from build123d import *

# Parameters (mm, degrees)
SKETCH_1_W             = 47.4
SKETCH_1_H             = 66.4
EXTRUDE_1_DEPTH        = 10
FILLET_1_R             = 3
FILLET_2_R             = 2
FILLET_4_R             = 1
FILLET_5_R             = 1
FILLET_1_OF_MIRROR_1_R = 3
FILLET_2_OF_MIRROR_1_R = 2
FILLET_4_OF_MIRROR_1_R = 1


with BuildPart() as part:
    # 草图1 → 凸台-拉伸1 (new body)
    with BuildSketch(Plane.XY):
        with BuildLine():
            ThreePointArc((-165.866679255, 23.5), (-260, 0), (-165.866679255, -23.5))
            Line((-165.866679255, -23.5), (0, -23.5))
            Line((0, -23.5), (0, 23.5))
            Line((0, 23.5), (-165.866679255, 23.5))
        make_face()
        with BuildLine():
            ThreePointArc((-187.901131251, -39.2), (-210, -45), (-232.098868749, -39.2))
            Line((-232.098868749, -39.2), (-187.901131251, -39.2))
        make_face(mode=Mode.SUBTRACT)
        with BuildLine():
            ThreePointArc((-239.7, -33.806951948), (-255, 0), (-239.7, 33.806951948))
            Line((-239.7, 33.806951948), (-239.7, -33.806951948))
        make_face(mode=Mode.SUBTRACT)
        with Locations((-210, 0)):
            Rectangle(SKETCH_1_W, SKETCH_1_H, mode=Mode.SUBTRACT)
        with BuildLine():
            Line((-187.901131251, 39.2), (-232.098868749, 39.2))
            ThreePointArc((-232.098868749, 39.2), (-210, 45), (-187.901131251, 39.2))
        make_face(mode=Mode.SUBTRACT)
    extrude_1 = extrude(amount=EXTRUDE_1_DEPTH)

    # 圆角1
    fillet_1_edges = [part.edges().sort_by_distance(p)[0] for p in [
        (-186.3, 33.2, 5),
        (-233.7, 33.2, 5),
        (-233.7, -33.2, 5),
        (-186.3, -33.2, 5),
    ]]
    fillet(fillet_1_edges, radius=FILLET_1_R)

    # 圆角2
    fillet_2_edges = [part.edges().sort_by_distance(p)[0] for p in [
        (-239.7, 33.806951948, 5),
        (-239.7, -33.806951948, 5),
    ]]
    fillet(fillet_2_edges, radius=FILLET_2_R)

    # 圆角4
    fillet_4_edges = [part.edges().sort_by_distance(p)[0] for p in [
        (-187.901131251, 39.2, 5),
        (-232.098868749, 39.2, 5),
        (-187.901131251, -39.2, 5),
        (-232.098868749, -39.2, 5),
    ]]
    fillet(fillet_4_edges, radius=FILLET_4_R)

    # 圆角5
    fillet_5_edges = [part.edges().sort_by_distance(p)[0] for p in [
        (-260, 0, 10),
        (-260, 0, 0),
    ]]
    fillet(fillet_5_edges, radius=FILLET_5_R)

    # 镜向1: 凸台-拉伸1 across plane
    add(extrude_1.mirror(Plane(origin=(0, 0, 10), x_dir=(0, 0, 1), z_dir=(1, 0, 0))))

    # 圆角1 of 镜向1
    fillet_1_of_mirror_1_edges = [part.edges().sort_by_distance(p)[0] for p in [
        (186.3, 33.2, 5),
        (233.7, 33.2, 5),
        (233.7, -33.2, 5),
        (186.3, -33.2, 5),
    ]]
    fillet(fillet_1_of_mirror_1_edges, radius=FILLET_1_OF_MIRROR_1_R)

    # 圆角2 of 镜向1
    fillet_2_of_mirror_1_edges = [part.edges().sort_by_distance(p)[0] for p in [
        (239.7, 33.806951948, 5),
        (239.7, -33.806951948, 5),
    ]]
    fillet(fillet_2_of_mirror_1_edges, radius=FILLET_2_OF_MIRROR_1_R)

    # 圆角4 of 镜向1
    fillet_4_of_mirror_1_edges = [part.edges().sort_by_distance(p)[0] for p in [
        (187.901131251, 39.2, 5),
        (232.098868749, 39.2, 5),
        (187.901131251, -39.2, 5),
        (232.098868749, -39.2, 5),
    ]]
    fillet(fillet_4_of_mirror_1_edges, radius=FILLET_4_OF_MIRROR_1_R)


solid = part.part
Geometry check sheet. Reference: the model listing, model coordinates, mm. A direction names the side the tool comes from. Give positions to 0.01 mm unless a question says otherwise; leave off trailing zeros. Order: outer loops, then holes, each group sorted by start corner. A loop starts at its lowest first (then second) coordinate and runs counter-clockwise, first axis right, second up. Notation, with made-up numbers: M 42,51.25 L 53,51.25 A8 cw 53,64.25 Z; hole C 16.5,-14 d11. An arc over 180 degrees is marked long. Use a Markdown table: item, result.
Item 1: Draft check along Y on faces 3 (the cylindrical face through (-259.966, 1.856, 4.944)), 4 (the flat face through (-186.3, 0, 5)), 5 (the flat face through (-239.7, 0, 5)), 6 (the flat face through (-3, 23.5, 5)). Enter one of: +Y half, -Y half, draft (parallel to the pull), parting line (faces both ways), or undercut.
Answers follow:
| item | result |
|---|---|
| face 3 | parting line |
| face 4 | undercut |
| face 5 | undercut |
| face 6 | +Y half |
Item 2: Depth check by flat-ended pin: P1, Ø4, axis at x = 48.5, z = 3, coming from the +Y side; P2, Ø3, axis at y = 12, z = 5.5, coming from the -X side; P3, Ø3, axis at y = 4.5, z = 5.5, coming from the -X side. Enter the tip coordinate at first touch or a pass-through.
Answers follow:
| item | result |
|---|---|
| P1 | stops at y = 23.5 |
| P2 | stops at x = -258.89 |
| P3 | stops at x = -259.91 |
Item 3: Section check B-B (x = 210). Record the cut outline in (y, z).
Answers follow:
| item | result |
|---|---|
| outline | M -50,0 L -45,0 L -45,10 L -50,10 Z; M -39.2,0 L -33.2,0 L -33.2,10 L -39.2,10 Z; M 33.2,0 L 39.2,0 L 39.2,10 L 33.2,10 Z; M 45,0 L 50,0 L 50,10 L 45,10 Z |
Item 4: Tool access check on faces 1 (the flat face through (4, 1, 0)), 2 (the flat face through (239.7, 0, 5)). Record the directions out of +Z, -Z, +X, -X, +Y, -Y that give a thin tool (end or side, any length) a straight path to the whole face; none if there is none.
Answers follow:
| item | result |
|---|---|
| face 1 | -Z, +X, -X, +Y, -Y |
| face 2 | +Z, -Z |
Item 5: Section check D-D (z = 4.5). State how many separate pieces and enclosed holes the cut face has, and give its area (3 significant figures).
Answers follow:
| item | result |
|---|---|
| separate pieces | 1 |
| enclosed holes | 8 |
| area | 22,600 mm2 |
Item 6: Section check C-C (x = -139). Record the cut outline in (y, z).
Answers follow:
| item | result |
|---|---|
| outline | M -23.5,0 L 23.5,0 L 23.5,10 L -23.5,10 Z |
Item 7: Section check A-A (y = 0). Record the cut outline in (x, z).
Answers follow:
| item | result |
|---|---|
| outline | M -260,1 A1 ccw -259,0 L -255,0 L -255,10 L -259,10 A1 ccw -260,9 Z; M -239.7,0 L -233.7,0 L -233.7,10 L -239.7,10 Z; M -186.3,0 L 186.3,0 L 186.3,10 L -186.3,10 Z; M 233.7,0 L 239.7,0 L 239.7,10 L 233.7,10 Z; M 255,0 L 260,0 L 260,10 L 255,10 Z |
Item 8: Material ranges on line 1 along X through (y, z) = (-1.5, 6.5) (1 decimal); line 2 along X through (y, z) = (-18.5, 7); line 3 along Y through (x, z) = (219, 5), recorded low to high.
Answers follow:
| item | result |
|---|---|
| line 1 | x = -260 to -255, -239.7 to -233.7, -186.3 to 186.3, 233.7 to 239.7, 255 to 260 |
| line 2 | x = -256.45 to -251.02, -239.7 to -233.7, -186.3 to 186.3, 233.7 to 239.7, 251.02 to 256.45 |
| line 3 | y = -49.18 to -44.09, -39.2 to -33.2, 33.2 to 39.2, 44.09 to 49.18 |
